Build history of the part. All positions in model axes, mm. A direction names the side the tool comes from. Round coordinates to 2 decimals unless told otherwise and drop trailing zeros. Write each loop counter-clockwise with the first axis right and the second up, starting at its lowest first coordinate (ties: lowest second). Pieces come first, ordered by that corner, then holes. Notation, with made-up numbers: (4, 54.25) - (15, 54.25) arc R27 ccw to (15, 92.25) - close; hole circle Ø6 at (84.5, -18.75). An arc over 180 degrees is marked (long way). One line per question, with ' | ' between items.
from build123d import *

# Parameters (mm, degrees)
F0_W = 12.7
F0_H = 11.90625


with BuildPart() as f1:
    # F0 (on Front) → F1 (revolve)
    with BuildSketch(Plane.XZ):
        with Locations((-31.75, 5.953125)):
            Rectangle(F0_W, F0_H)
        with BuildLine():
            Line((-25.4, 11.90625), (-25.4, 0))
            Line((-25.4, 0), (0, 0))
            Line((0, 0), (0, 11.90625))
            Line((0, 11.90625), (0, 25.4))
            Line((0, 25.4), (-1.480527, 22.225))
            ThreePointArc((-1.480527, 22.225), (-12.7, 11.005527), (-23.919473, 22.225))
            Line((-23.919473, 22.225), (-25.4, 25.4))
            Line((-25.4, 25.4), (-25.4, 11.90625))
        make_face()
        with Locations((6.35, 5.953125)):
            Rectangle(F0_W, F0_H)
    revolve(axis=Axis((-11.84914, 0, 0), (1, 0, 0)))


solid = f1.part
Q1. Pull direction X, two halves, no side cores. Call faces 1 (the conical face through (-1.409, 21.847, -4.851)), 2 (the flat face through (-25.4, 5, 11)), 3 (the flat face through (12.7, 0, 0)): +X half, -X half, draft (parallel to the pull), parting line (faces both ways), or undercut.
Found:
face 1: undercut | face 2: -X half | face 3: +X half
Q2. Saw through at A-A, the plane y = 0. List the corners of the cut face in (x, z) (3 decimals), then the cut area to 3 significant figures.
Found:
outline: (-38.1, -11.906) - (-25.4, -11.906) - (-25.4, -25.4) - (-23.919, -22.225) arc R11.219 cw to (-1.481, -22.225) - (0, -25.4) - (0, -11.906) - (12.7, -11.906) - (12.7, 11.906) - (0, 11.906) - (0, 25.4) - (-1.481, 22.225) arc R11.219 cw to (-23.919, 22.225) - (-25.4, 25.4) - (-25.4, 11.906) - (-38.1, 11.906) - close | area: 1,350 mm^2
Q3. Drill centre lines: L1, parallel to X at y = -8.5, z = -9; L2, parallel to X at y = 0, z = 16; L3, parallel to Z at x = -36, y = -7.5. Where is each one in solid material? Low to high. Write a range as from..to.
Found:
L1: -25.4..-18.08, -7.32..0 | L2: -25.4..-22.03, -3.37..0 | L3: -9.25..9.25
Q4. Saw through at D-D, the plane x = -10. List the corners of the cut face in (y, z), then the cut area to 3 significant figures.
Found:
outline: circle Ø22.67 at (0, 0) | area: 404 mm^2
Q5. Saw through at C-C, the plane x = 3.5. List the corners of the cut face in (y, z), then the cut area to 3 significant figures.
Found:
outline: circle Ø23.81 at (0, 0) | area: 445 mm^2
Q6. Which spindle directions (+Z, -Z, +X, -X, +Y, -Y) get a long thin tool onto all of the face, cutting with end or side? Do faces 4 (the flat face through (-38.1, 0, 0)), 5 (the conical face through (-24.01, 21.89, -4.86)), 6 (the cylindrical face through (-31.66, 7.24, -9.45)), 7 (the cylindrical face through (6.44, 7.24, -9.45)). Say none if no direction does.
Found:
face 4: +Z, -Z, -X, +Y, -Y | face 5: none | face 6: -X | face 7: +X
Q7. Drop flat-ended pins along their axis: pin 1 (1 mm diameter, centred on y = -15.5, z = 18.5, fed in from +X); pin 2 (5 mm diameter, centred on x = -5, y = -19.5, fed in from -Z); pin 3 (5 mm diameter, centred on x = -22, z = 2, fed in from -Y). Give the stop position or say it passes through.
Found:
pin 1: x = 0 | pin 2: through | pin 3: y = -23.39
